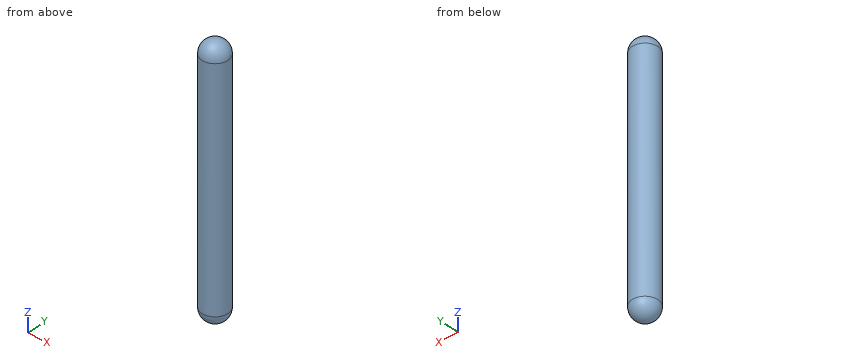
Autodesk Inventor part; units mm, degrees
ref_plane "YZ Plane" through (0, 0, 0) normal (1, 0, 0) x (0, 1, 0)
ref_plane "XZ Plane" through (0, 0, 0) normal (0, 1, 0) x (-1, 0, 0)
ref_plane "XY Plane" through (0, 0, 0) normal (0, 0, 1) x (1, 0, 0)
sketch "Sketch1" plane through (0, 0, 0) normal (0, 0, 1) x (1, 0, 0)
  circle A0 centre (0, 0) radius 2
  dimension "d6" = 4
extrude "Extrusion2" add sketch "Sketch1" along normal blind 40
fillet "Fillet4" radius 2 2 edges at (-2, 0, 0) (-2, 0, 40)
scale "Scale1" factors (0.5, 0.5, 0.5) then translate (0, 0, 10) bodies 1
properties part number "Pasador"
Here's how the part is built. I have some questions about the finished solid (model axes, mm). Round coordinates to 2 decimals unless told otherwise and drop trailing zeros. Order: outer loops, then holes, each group sorted by start corner. A loop starts at its lowest first (then second) coordinate and runs counter-clockwise, first axis right, second up. Notation, with made-up numbers: M 14.25,30.5 L 51.25,30.5 A23 ccw 51.25,67.5 Z; hole C -9.75,-26.5 d8. An arc over 180 degrees is marked long. One line per question, with ' | ' between items.
1) I want a section at A-A, the plane y = 0. Write out the boundary of the cut face in (x, z), then the cut area to 3 significant figures.
Working result:
outline: M -1,11 A1 ccw 1,11 L 1,29 A1 ccw -1,29 Z | area: 39.1 mm²
2) I need wall thicknesses on line 1 along Z through (x, y) = (0.05, 0); line 2 along Z through (x, y) = (0.75, -0.4); line 3 along Y through (x, z) = (0.3, 23.25). Which ranges of each line are inside material? Lowest first, please.
Working result:
line 1: 10 to 30 | line 2: 10.47 to 29.53 | line 3: -0.95 to 0.95
3) I want a section at C-C, the plane z = 23.25. Write out the boundary of the cut face in (x, y).
Working result:
outline: C 0,0 d2
